Design review of the part built by this model. Coordinates are the model's own, in mm. A direction names the side the tool comes from. Round coordinates to 2 decimals unless told otherwise and drop trailing zeros. Write each loop counter-clockwise with the first axis right and the second up, starting at its lowest first coordinate (ties: lowest second). Pieces come first, ordered by that corner, then holes. Notation, with made-up numbers: (-5.5, 79) - (6.5, 79) arc R35 ccw to (6.5, 118) - close; hole circle Ø10 at (-37.75, -33.75). An arc over 180 degrees is marked (long way). Use one line per item in the form item = value.
```python
from build123d import *

# Parameters (mm, degrees)
F3_SIZE2 = 2.9329393675
F3_SIZE  = 5.08


# Not quite as in the source:
# - a fillet or chamfer that OpenCascade refuses, or shapes differently, is made with other operations: its cross-section is extruded or revolved along the edge and cut away or added


with BuildPart() as f1:
    # F0 (on Front) → F1 (revolve)
    with BuildSketch(Plane.XZ):
        Polygon((3.175, 44.45), (0, 44.45), (0, 0), (50.8, 0), (50.8, 12.7), (25.478093854, 12.7), (25.4, 12.7), (25.4, 2.54), (3.175, 2.54), align=None)
        Polygon((50.8, 0), (0, 0), (0, -44.45), (3.175, -44.45), (3.175, -2.54), (25.4, -2.54), (25.4, -12.7), (50.8, -12.7), align=None)
    revolve(axis=Axis((0, 0, 0), (0, 0, 1)))

    # F2: chamfer of 5.08 x 2.9329393675 on 1 edges, made by hand

    # F2_s1 → F2_t2 (revolve, cut)
    with BuildSketch(Plane.XZ):
        Polygon((3.175, 39.37), (0.2420606325, 44.45), (3.175, 44.45), align=None)
    revolve(axis=Axis((0, 0, 44.45), (0, 0, 1)), mode=Mode.SUBTRACT)

    # F3
    f3_edges = [f1.edges().sort_by_distance(p)[0] for p in [
        (-3.175, 0, -44.45),
    ]]
    chamfer(f3_edges, length=F3_SIZE, length2=F3_SIZE2)

    # F4 (on Front) → F5 (revolve)
    with BuildSketch(Plane.XZ):
        with BuildLine():
            Line((50.8, -12.7), (54.4176846255, -12.7))
            ThreePointArc((54.4176846255, -12.7), (55.88, 0), (54.4176846255, 12.7))
            Line((54.4176846255, 12.7), (50.8, 12.7))
            Line((50.8, 12.7), (50.8, -12.7))
        make_face()
    revolve(axis=Axis((0, 0, 12.7), (0, 0, 1)))


solid = f1.part
```
Q1. We need section A-A on z = 7. Write out the cut boundary in (x, y) (3 decimals).
Calculated:
outline = circle Ø110.88 at (0, 0); circle Ø6.35 at (0, 0); hole circle Ø50.8 at (0, 0)
Q2. We need section C-C on z = 29.5. Write out the cut boundary in (x, y) (3 decimals).
Calculated:
outline = circle Ø6.35 at (0, 0)
Q3. Draft analysis for pull direction X (two halves, no side actions). For faces 3 (the flat face through (-23.4, -11.3, -12.7)), 4 (the conical face through (-0.18, 1.35, -42.51)), 5 (the cylindrical face through (-5.506, -24.796, -7.691)), state which applies: released by +X, released by -X, zero draft, split by the parting line, or undercut.
Calculated:
face_3 = zero draft
face_4 = split by the parting line
face_5 = undercut
Q4. Machinability: for faces 1 (the flat face through (-5, 0, -2.54)), 2 (the cylindrical face through (-0.69, -3.1, 21.21)), which of the approach directions +Z, -Z, +X, -X, +Y, -Y give a long, thin tool a straight path to every point of the face, cutting with its end or side? Answer none if there is none.
Calculated:
face_1 = -Z
face_2 = +Z
Q5. We need section D-D on x = 11. Write out the cut boundary in (y, z), then the cut area to 3 significant figures.
Calculated:
outline = (-53.29, -12.7) - (-22.89, -12.7) - (-22.89, -2.54) - (22.89, -2.54) - (22.89, -12.7) - (53.29, -12.7) arc R54.79 ccw to (53.29, 12.7) - (22.89, 12.7) - (22.89, 2.54) - (-22.89, 2.54) - (-22.89, 12.7) - (-53.29, 12.7) arc R54.79 ccw to start
area = 1,830 mm2
Q6. We need section B-B on y = 21.5. Write out the cut boundary in (x, z), then the cut area to 3 significant figures.
Calculated:
outline = (-49.99, -12.7) - (-13.52, -12.7) - (-13.52, -2.54) - (13.52, -2.54) - (13.52, -12.7) - (49.99, -12.7) arc R51.58 ccw to (49.99, 12.7) - (13.52, 12.7) - (13.52, 2.54) - (-13.52, 2.54) - (-13.52, 12.7) - (-49.99, 12.7) arc R51.58 ccw to start
area = 2,040 mm2
Q7. For P1, Ø1, axis at x = -30.5, y = -41, coming from the +Z side; P2, Ø1.5, axis at x = 40, y = 18.5, coming from the -Z side; P3, Ø8, axis at y = 4.5, z = -28.5, coming from the -X side; P4, Ø6, axis at x = -7.5, z = -28, coming from the +Y side, all flat-tipped, find the tip position at first contact; note any pin that passes through.
Calculated:
P1 = 12.7
P2 = -12.7
P3 = -3.14
P4 = through
Q8. To check wall thickness, follow line 1 along Y through (x, z) = (0, 10) (3 decimals); line 2 along Z through (x, y) = (12.5, -21); line 3 along Z through (x, y) = (-6, -43.5). State the ranges of each line that lie inside material, in increasing order. Write a range as from..to.
Calculated:
line_1 = -54.978..-25.4, -3.175..3.175, 25.4..54.978
line_2 = -2.54..2.54
line_3 = -12.7..12.7
